Could you check a few things on this model? Use its own coordinates, in mm. A direction names the side the tool comes from. Coordinates: 2 decimals unless noted, no trailing zeros. Order: outer loops, then holes, each group sorted by start corner. A loop starts at its lowest first (then second) coordinate and runs counter-clockwise, first axis right, second up. Notation, with made-up numbers: (40, -22.5) -> (51, -22.5) arc R11 cw to (51, -1.5) -> close; hole circle Ø4 at (83, 39.25). An arc over 180 degrees is marked (long way). Return JSON: item names as keys, results as strings. Group by question number.
from build123d import *
from build123d.topology import SkipClean

# Parameters (mm, degrees)
BOSS_EXTRUDE1_DEPTH = 3.5
BOSS_EXTRUDE2_START = 1.75
SKETCH3_R           = 3.5
BOSS_EXTRUDE2_DEPTH = 1.75
BOSS_EXTRUDE3_START = 1.75
SKETCH3_3_R         = 5
BOSS_EXTRUDE3_DEPTH = 0.5
SKETCH4_R           = 3
CUT_EXTRUDE2_DEPTH  = 8.25
SKETCH5_R           = 0.75
CUT_EXTRUDE3_DEPTH  = 8.25
BOSS_EXTRUDE4_DEPTH = 8.25
CUT_EXTRUDE4_REACH  = 18.856
SKETCH7_R           = 0.375


with BuildPart() as part:
    # Sketch1 → Boss-Extrude1 (new, symmetric)
    with BuildSketch(Plane.XY):
        with BuildLine():
            Line((-6, 0), (6, 0))
            Line((6, 0), (3.312648335, 7.879761483))
            ThreePointArc((3.312648335, 7.879761483), (0, 10.25), (-3.312648335, 7.879761483))
            Line((-3.312648335, 7.879761483), (-6, 0))
        make_face()
    extrude(amount=BOSS_EXTRUDE1_DEPTH, both=True)

    # Sketch3 → Boss-Extrude2 (add)
    with SkipClean():  # the faces are left unmerged after this step: merging them gives an invalid solid
        with BuildSketch(Plane.XY.offset(3.5).offset(BOSS_EXTRUDE2_START)):
            with Locations(Location((0, 6.75, 0), (0, 0, 161.168324383))):
                Circle(SKETCH3_R)
        extrude(amount=-BOSS_EXTRUDE2_DEPTH)

    # Sketch3<3> → Boss-Extrude3 (add)
    with BuildSketch(Plane.XY.offset(3.5).offset(BOSS_EXTRUDE3_START)):
        with Locations((0, 6.75)):
            Circle(SKETCH3_3_R)
    extrude(amount=BOSS_EXTRUDE3_DEPTH)

    # Sketch4 → Cut-Extrude2 (cut)
    with SkipClean():  # the faces are left unmerged after this step: merging them gives an invalid solid
        with BuildSketch(Plane.XY.offset(5.75)):
            with Locations((0, 6.75)):
                Circle(SKETCH4_R)
        extrude(amount=-CUT_EXTRUDE2_DEPTH, mode=Mode.SUBTRACT)

    # Sketch5 → Cut-Extrude3 (cut)
    with SkipClean():  # the faces are left unmerged after this step: merging them gives an invalid solid
        with BuildSketch(Plane(origin=(0, 0, -3.5), x_dir=(-1, 0, 0), z_dir=(0, 0, -1))):
            with Locations((0, 6.75)):
                Circle(SKETCH5_R)
        extrude(amount=-CUT_EXTRUDE3_DEPTH, mode=Mode.SUBTRACT)

    # Sketch6 → Boss-Extrude4 (add)
    with SkipClean():  # the faces are left unmerged after this step: merging them gives an invalid solid
        with BuildSketch(Plane(origin=(0, 0, 5.25), x_dir=(-1, 0, 0), z_dir=(0, 0, -1))):
            with BuildLine():
                Line((3, 12.75), (-3, 12.75))
                Line((-3, 12.75), (-3, 12.3075))
                Line((-3, 12.3075), (-2.5, 12.3075))
                Line((-2.5, 12.3075), (-2.5, 11.8575))
                Line((-2.5, 11.8575), (-3, 11.8575))
                Line((-3, 11.8575), (-3, 11.415))
                Line((-3, 11.415), (-2.5, 11.415))
                Line((-2.5, 11.415), (-2.5, 10.965))
                Line((-2.5, 10.965), (-3, 10.965))
                Line((-3, 10.965), (-3, 10.5225))
                Line((-3, 10.5225), (-2.5, 10.5225))
                Line((-2.5, 10.5225), (-2.5, 10.0725))
                Line((-2.5, 10.0725), (-3, 10.0725))
                Line((-3, 10.0725), (-3, 9.63))
                Line((-3, 9.63), (-2.5, 9.63))
                Line((-2.5, 9.63), (-2.5, 9.199489743))
                ThreePointArc((-2.5, 9.199489743), (0, 10.25), (2.5, 9.199489743))
                Line((2.5, 9.199489743), (2.5, 9.63))
                Line((2.5, 9.63), (3, 9.63))
                Line((3, 9.63), (3, 10.0725))
                Line((3, 10.0725), (2.5, 10.0725))
                Line((2.5, 10.0725), (2.5, 10.5225))
                Line((2.5, 10.5225), (3, 10.5225))
                Line((3, 10.5225), (3, 10.965))
                Line((3, 10.965), (2.5, 10.965))
                Line((2.5, 10.965), (2.5, 11.415))
                Line((2.5, 11.415), (3, 11.415))
                Line((3, 11.415), (3, 11.8575))
                Line((3, 11.8575), (2.5, 11.8575))
                Line((2.5, 11.8575), (2.5, 12.3075))
                Line((2.5, 12.3075), (3, 12.3075))
                Line((3, 12.3075), (3, 12.75))
            make_face()
            with BuildLine():
                Line((3, 9.18), (2.518948193, 9.18))
                ThreePointArc((2.518948193, 9.18), (2.777237817, 8.880011763), (3, 8.552775638))
                Line((3, 8.552775638), (3, 9.18))
            make_face()
            with BuildLine():
                ThreePointArc((-3, 8.552775638), (-2.777237817, 8.880011763), (-2.518948193, 9.18))
                Line((-2.518948193, 9.18), (-3, 9.18))
                Line((-3, 9.18), (-3, 8.552775638))
            make_face()
        extrude(amount=BOSS_EXTRUDE4_DEPTH)

    # Sketch7 → Cut-Extrude4 (cut, up to next)
    with BuildSketch(Plane.XY.offset(5.75), mode=Mode.PRIVATE) as cut_extrude4_sk1:
        with Locations((0, 2.5)):
            Circle(SKETCH7_R)
    cut_extrude4_tool1 = extrude(cut_extrude4_sk1.sketch, amount=-CUT_EXTRUDE4_REACH, mode=Mode.PRIVATE) & part.part
    # Sketch7 → Cut-Extrude4 (cut, up to next)
    with BuildSketch(Plane.XY.offset(5.75), mode=Mode.PRIVATE) as cut_extrude4_sk2:
        with Locations((3.680607966, 8.875)):
            Circle(SKETCH7_R)
    cut_extrude4_tool2 = extrude(cut_extrude4_sk2.sketch, amount=-CUT_EXTRUDE4_REACH, mode=Mode.PRIVATE) & part.part
    # Sketch7 → Cut-Extrude4 (cut, up to next)
    with BuildSketch(Plane.XY.offset(5.75), mode=Mode.PRIVATE) as cut_extrude4_sk3:
        with Locations((-3.680607966, 8.875)):
            Circle(SKETCH7_R)
    cut_extrude4_tool3 = extrude(cut_extrude4_sk3.sketch, amount=-CUT_EXTRUDE4_REACH, mode=Mode.PRIVATE) & part.part
    add(cut_extrude4_tool1.solids().sort_by_distance((0, 2.5, 5.75))[0], mode=Mode.SUBTRACT)
    add(cut_extrude4_tool2.solids().sort_by_distance((3.680608, 8.875, 5.75))[0], mode=Mode.SUBTRACT)
    add(cut_extrude4_tool3.solids().sort_by_distance((-3.680608, 8.875, 5.75))[0], mode=Mode.SUBTRACT)


solid = part.part
Q1. On a 3-axis mill with a long thin cutter (end or side, diameter ignored), from which of +Z, -Z, +X, -X, +Y, -Y can I reach the whole of each face in a straight line? I mean faces 4 (the flat face through (-4.638, 3.995, 0.049)), 5 (the flat face through (4.675, 3.885, 0.049)), 6 (the flat face through (1, 6, -2.5)). Say none if no direction works.
Q2. I want a section at D-D on y = 2.5. Please give me the cut outline in (x, z) (3 decimals).
Q3. I want a section at B-B on y = 6.75. Please give me the cut outline in (x, z), and give its area (3 significant figures).
Q4. I'm going to push flat-ended pins straight in: pin 1 Ø0.5 at (y, z) = (11, 0.5) entering from -X; pin 2 Ø2 at (y, z) = (6, 1) entering from -X; pin 3 Ø1 at (y, z) = (3.5, -1) entering from +X. Where does each tip first touch, or does it pass through?
Q5. I want a section at A-A on x = 0. Please give me the cut outline in (y, z) (3 decimals), and give its area (4 significant figures).
Q6. I need wall thicknesses on line 1 along Z through (x, y) = (-1.5, 6.75); line 2 along X through (y, z) = (11.25, -0.25); line 3 along Y through (x, z) = (1.75, -0.5). Which ranges of each line are inside material? Lowest first, please. Write a range as from..to.
Q7. I want a section at C-C on y = 5. Please give me the cut outline in (x, z).
Q8. We'd pull the mould along Z, two halves only. Please class faces 1 (the flat face through (0, 4, -3.5)), 2 (the flat face through (0, 2, 3.5)), 3 (the flat face through (0, 12.75, 1)): pulls with the +Z half, pulls with the -Z half, needs draft (parallel to the pull), parting line crosses it, or undercut.
Response values:
{
 "1": {"face 4": "-Z, -X, +Y", "face 5": "-Z, +X, +Y", "face 6": "+Z"},
 "2": {"outline": "(-5.147, -3.5) -> (5.147, -3.5) -> (5.147, 3.5) -> (-5.147, 3.5) -> close; (-2.634, 5.25) -> (-0.375, 5.25) -> (-0.375, 5.75) -> (-2.634, 5.75) -> close; (0.375, 5.25) -> (2.634, 5.25) -> (2.634, 5.75) -> (0.375, 5.75) -> close"},
 "3": {"outline": "(-5, 5.25) -> (-3.5, 5.25) -> (-3.5, 3.5) -> (-3.7, 3.5) -> (-3.7, -3.5) -> (-0.75, -3.5) -> (-0.75, -2.5) -> (-3, -2.5) -> (-3, 5.75) -> (-5, 5.75) -> close; (0.75, -3.5) -> (3.7, -3.5) -> (3.7, 3.5) -> (3.5, 3.5) -> (3.5, 5.25) -> (5, 5.25) -> (5, 5.75) -> (3, 5.75) -> (3, -2.5) -> (0.75, -2.5) -> close", "area": "18.0 mm²"},
 "4": {"pin 1": "stops at x = -3", "pin 2": "stops at x = -4.29", "pin 3": "stops at x = 4.98"},
 "5": {"outline": "(0, -3.5) -> (6, -3.5) -> (6, -2.5) -> (3.75, -2.5) -> (3.75, 5.75) -> (2.875, 5.75) -> (2.875, 5.25) -> (3.25, 5.25) -> (3.25, 3.5) -> (0, 3.5) -> close; (1.75, 5.25) -> (2.125, 5.25) -> (2.125, 5.75) -> (1.75, 5.75) -> close; (7.5, -3.5) -> (10.25, -3.5) -> (10.25, -3) -> (12.75, -3) -> (12.75, 5.25) -> (11.75, 5.25) -> (11.75, 5.75) -> (9.75, 5.75) -> (9.75, -2.5) -> (7.5, -2.5) -> close", "area": "58.25 mm²"},
 "6": {"line 1": "z = -3.5..-2.5", "line 2": "x = -2.5..2.5", "line 3": "y = 0..4.31, 9.19..12.75"},
 "7": {"outline": "(-4.68, 5.25) -> (-3.03, 5.25) -> (-3.03, 3.5) -> (-4.29, 3.5) -> (-4.29, -3.5) -> (4.29, -3.5) -> (4.29, 3.5) -> (3.03, 3.5) -> (3.03, 5.25) -> (4.68, 5.25) -> (4.68, 5.75) -> (2.44, 5.75) -> (2.44, -2.5) -> (-2.44, -2.5) -> (-2.44, 5.75) -> (-4.68, 5.75) -> close"},
 "8": {"face 1": "pulls with the -Z half", "face 2": "undercut", "face 3": "needs draft"}
}
